Geometry check sheet. Reference: the model listing, model coordinates, mm. Coordinates: 2 decimals unless noted, no trailing zeros. Order: outer loops, then holes, each group sorted by start corner. A loop starts at its lowest first (then second) coordinate and runs counter-clockwise, first axis right, second up. Notation, with made-up numbers: (70.5, -14) - (87.5, -14) arc R29 cw to (87.5, 23) - close; hole circle Ø3 at (87, -0.75). An arc over 180 degrees is marked (long way). Put each result on its own line as item: value.
from build123d import *

# Parameters (mm, degrees)
SKETCH_1_W      = 25
SKETCH_1_H      = 5
EXTRUDE_1_DEPTH = 5
FILLET_1_R      = 100


with BuildPart() as part:
    # 草图1 → 凸台-拉伸1 (new body)
    with BuildSketch(Plane.XY):
        Polygon((-40, 0), (-34.5, 0), (-34.5, 6), (-36, 6), (-36, 8.9), (-34.5, 8.9), (-34.5, 11), (-30.5, 11), (-30.5, 8.9), (-29, 8.9), (-29, 6), (-30.5, 6), (-30.5, 0), (0, 0), (0, 20), (-15, 20), (-65, 16), (-115, 20), (-130, 20), (-130, 0), (-99.5, 0), (-99.5, 6), (-101, 6), (-101, 8.9), (-99.5, 8.9), (-99.5, 11), (-95.5, 11), (-95.5, 8.9), (-94, 8.9), (-94, 6), (-95.5, 6), (-95.5, 0), (-90, 0), (-90, -5), (-40, -5), align=None)
        with Locations((-65, 10.5)):
            Rectangle(SKETCH_1_W, SKETCH_1_H, mode=Mode.SUBTRACT)
    extrude(amount=EXTRUDE_1_DEPTH)

    # 圆角1
    fillet_1_edges = [part.edges().sort_by_distance(p)[0] for p in [
        (-65, 16, 2.5),
    ]]
    fillet(fillet_1_edges, radius=FILLET_1_R)


solid = part.part
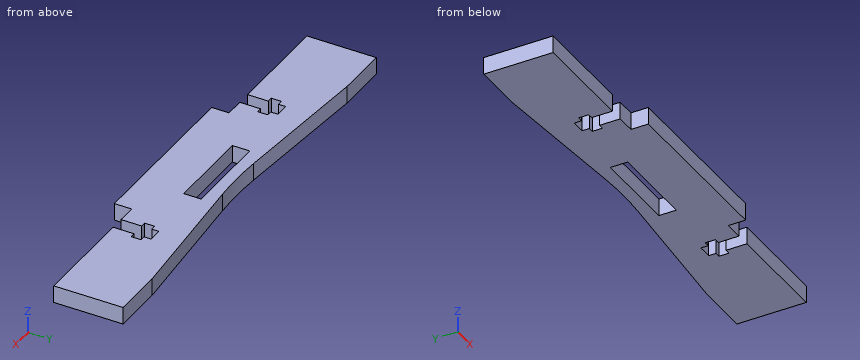
Q1. Section check A-A on y = 18.25. Record the boundary of the cut face in (x, z) (3 decimals), then the cut area to 3 significant figures.
Answer block:
outline: (-130, 0) - (-93.125, 0) - (-93.125, 5) - (-130, 5) - close; (-36.875, 0) - (0, 0) - (0, 5) - (-36.875, 5) - close
area: 369 mm^2
Q2. Section check C-C on y = -3.25. Record the boundary of the cut face in (x, z), then the cut area to 3 significant figures.
Answer block:
outline: (-90, 0) - (-40, 0) - (-40, 5) - (-90, 5) - close
area: 250 mm^2
Q3. Section check B-B on x = -86. Record the boundary of the cut face in (y, z), then the cut area to 3 significant figures.
Answer block:
outline: (-5, 0) - (17.68, 0) - (17.68, 5) - (-5, 5) - close
area: 113 mm^2
Q4. Thickness scan on L1, parallel to X at y = 7.5, z = 0.8; L2, parallel to X at y = 9, z = 1.35; L3, parallel to X at y = 4.25, z = 3.3. Record the ranges inside material, lowest first. Write a range as [from, to].
Answer block:
L1: x = [-130, -101], [-94, -36], [-29, 0]
L2: x = [-130, -99.5], [-95.5, -77.5], [-52.5, -34.5], [-30.5, 0]
L3: x = [-130, -99.5], [-95.5, -34.5], [-30.5, 0]
Q5. Depth check by flat-ended pin: pin 1 Ø1.6 at (x, z) = (-100.5, 2) entering from +Y; pin 2 Ø3 at (x, z) = (-97.5, 1.5) entering from -Y; pin 3 Ø2 at (x, z) = (-50.5, 1) entering from +Y. Enter the tip coordinate at first touch or a pass-through.
Answer block:
pin 1: stops at y = 18.9
pin 2: stops at y = 11
pin 3: stops at y = 17.24
